Part model, mm, in its own coordinate system. Face numbers are marked on the shaded views. A direction names the side the tool comes from. Coordinates: 2 decimals unless noted, no trailing zeros. Loops run counter-clockwise (first coordinate to the right, second up) from the corner with the lowest first, then second, coordinate; pieces in that order, holes last. Notation, with made-up numbers: M 43.25,32 L 84.25,32 A28 cw 84.25,62 Z; hole C 14,50.25 d3. An arc over 180 degrees is marked long. Use a Markdown table: item, result. Add a question column.
1) Pull direction X, two halves, no side cores. Call the marked faces 1, 2, 3 and 4: released by +X, released by -X, zero draft, split by the parting line, or undercut.
2) Band-saw the part on D-D (x = 0.5). List the corners of the cut face in (y, z) (3 decimals).
3) Wall check: probe 1 along X at (y, z) = (0.25, -4); probe 2 along Z at (x, y) = (4, -4.75); probe 3 along Y at (x, z) = (4.75, 3.5). Give the ranges that are in metal, low to high. Write a range as from..to.
4) Pin check, flat tips, straight feed: pin 1 Ø3 at (x, z) = (-1, 1) entering from +Y; pin 2 Ø0.9 at (y, z) = (7.5, -3) entering from -X; pin 3 Ø1.5 at (y, z) = (0.5, -4) entering from +X. Stop position of each tip, or through.
5) Band-saw the part on B-B (z = -3). List the corners of the cut face in (x, y), plus the area to 3 significant figures.
6) Tool access for the marked faces 5, 6, 7 and 8: list every direction of +Z, -Z, +X, -X, +Y, -Y with a clear straight run to the whole face (end or side of a thin tool).
7) Band-saw the part on A-A (y = 11). List the corners of the cut face in (x, z), plus the area to 3 significant figures.
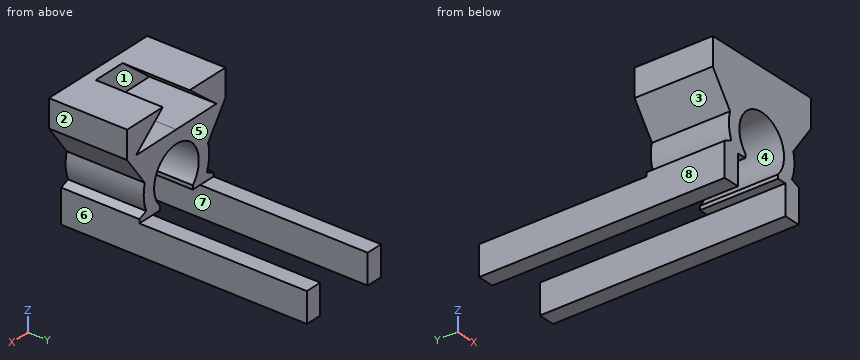
from build123d import *

# Parameters (mm, degrees)
F1_DEPTH = 7
F2_DEPTH = 6
F3_DEPTH = 15


with BuildPart() as f1:
    # F0 (on Front) → F1 (new body)
    with BuildSketch(Plane.XZ):
        with BuildLine():
            ThreePointArc((-3.477884, 0.719832), (-3.596369, -0.44229), (-3.343322, -1.5827))
            Line((-3.343322, -1.5827), (-3.322458, -1.593981))
            Line((-3.322458, -1.593981), (-3.322458, -2.283465))
            Line((-3.322458, -2.283465), (-2.589551, -2.283465))
            Line((-2.589551, -2.283465), (-1.76338, -2.283465))
            Line((-1.76338, -2.283465), (-1.76338, -1.934508))
            ThreePointArc((-1.76338, -1.934508), (0.063946, 2.271621), (1.891273, -1.934508))
            Line((1.891273, -1.934508), (1.891273, -2.283465))
            Line((1.891273, -2.283465), (2.717444, -2.283465))
            Line((2.717444, -2.283465), (3.450351, -2.283465))
            Line((3.450351, -2.283465), (3.450351, -1.634055))
            ThreePointArc((3.450351, -1.634055), (3.72254, -0.469953), (3.605777, 0.719832))
            ThreePointArc((3.605777, 0.719832), (2.307299, 2.6718), (0.091662, 3.438077))
            ThreePointArc((0.091662, 3.438077), (-2.157419, 2.688675), (-3.477884, 0.719832))
        make_face()
        Polygon((-3.322458, -2.283465), (-3.322458, -1.593981), (-4.089551, -1.943924), (-4.089551, -2.283465), align=None)
        with BuildLine():
            Line((-5.413338, 3.472093), (-3.477884, 0.719832))
            ThreePointArc((-3.477884, 0.719832), (-2.157419, 2.688675), (0.091662, 3.438077))
            Line((0.091662, 3.438077), (-4.408209, 3.472093))
            Line((-4.408209, 3.472093), (-1.413338, 5.938077))
            Line((-1.413338, 5.938077), (-5.413338, 5.938077))
            Line((-5.413338, 5.938077), (-5.413338, 3.472093))
        make_face()
        Polygon((-2.589551, -2.283465), (-3.322458, -2.283465), (-4.089551, -2.283465), (-4.089551, -4.949721), (-3.322458, -4.949721), (-2.589551, -4.949721), align=None)
        with BuildLine():
            Line((4.591534, 3.404061), (0.091662, 3.438077))
            ThreePointArc((0.091662, 3.438077), (2.307299, 2.6718), (3.605777, 0.719832))
            Line((3.605777, 0.719832), (5.587751, 3.472093))
            Line((5.587751, 3.472093), (5.587751, 5.938077))
            Line((5.587751, 5.938077), (1.596662, 5.938077))
            Line((1.596662, 5.938077), (4.591534, 3.404061))
        make_face()
        Polygon((-4.408209, 3.472093), (0.091662, 3.438077), (4.591534, 3.404061), (1.596662, 5.938077), (-1.413338, 5.938077), align=None)
        Polygon((4.217444, -1.943924), (3.450351, -1.634055), (3.450351, -2.283465), (4.217444, -2.283465), align=None)
        Polygon((4.217444, -2.283465), (3.450351, -2.283465), (2.717444, -2.283465), (2.717444, -4.949721), (3.450351, -4.949721), (4.217444, -4.949721), align=None)
    extrude(amount=F1_DEPTH)

    # F0 (on Front) → F2 (cut)
    with BuildSketch(Plane.XZ):
        Polygon((-4.408209, 3.472093), (0.091662, 3.438077), (4.591534, 3.404061), (1.596662, 5.938077), (-1.413338, 5.938077), align=None)
    extrude(amount=F2_DEPTH, mode=Mode.SUBTRACT)

    # F0 (on Front) → F3 (join)
    with BuildSketch(Plane.XZ):
        Polygon((4.217444, -2.283465), (3.450351, -2.283465), (2.717444, -2.283465), (2.717444, -4.949721), (3.450351, -4.949721), (4.217444, -4.949721), align=None)
        Polygon((-2.589551, -2.283465), (-3.322458, -2.283465), (-4.089551, -2.283465), (-4.089551, -4.949721), (-3.322458, -4.949721), (-2.589551, -4.949721), align=None)
    extrude(amount=-F3_DEPTH)


solid = f1.part
Entries:
| question | item | result |
|---|---|---|
| 1 | face 1 | undercut |
| 1 | face 2 | released by +X |
| 1 | face 3 | released by -X |
| 1 | face 4 | undercut |
| 2 | outline | M -7,2.233 L 0,2.233 L 0,3.435 L -6,3.435 L -6,5.938 L -7,5.938 Z |
| 3 | probe 1 | -4.09..-2.59, 2.72..4.22 |
| 3 | probe 2 | -4.95..-1.86, 1.27..3.41, 3.9..5.94 |
| 3 | probe 3 | -7..0 |
| 4 | pin 1 | y = 0 |
| 4 | pin 2 | x = -4.09 |
| 4 | pin 3 | x = 4.22 |
| 5 | outline | M -4.09,-7 L -2.59,-7 L -2.59,15 L -4.09,15 Z; M 2.72,-7 L 4.22,-7 L 4.22,15 L 2.72,15 Z |
| 5 | area | 66.0 mm2 |
| 6 | face 5 | +Z, +X, -X, +Y |
| 6 | face 6 | -Z, +X, +Y, -Y |
| 6 | face 7 | -Z, +Y, -Y |
| 6 | face 8 | -Z, -X, +Y, -Y |
| 7 | outline | M -4.09,-4.95 L -2.59,-4.95 L -2.59,-2.28 L -4.09,-2.28 Z; M 2.72,-4.95 L 4.22,-4.95 L 4.22,-2.28 L 2.72,-2.28 Z |
| 7 | area | 8.00 mm2 |
